Input: dimensioned drawing with shaded views. Units: mm. Origin: part minimum x, y, z. A direction names the side the tool comes from. Round coordinates to 2 decimals unless told otherwise and drop trailing zeros. Loops run counter-clockwise (first coordinate to the right, second up) from the corner with the lowest first, then second, coordinate; pieces in that order, holes last. Notation, with made-up numbers: (4.5, -35.5) -> (10.5, -35.5) arc R13 ccw to (10.5, -18.5) -> close; hole circle Ø3 at (48, 67.5). An arc over 180 degrees is marked (long way). Answer as a JSON object with one key per item and string values.
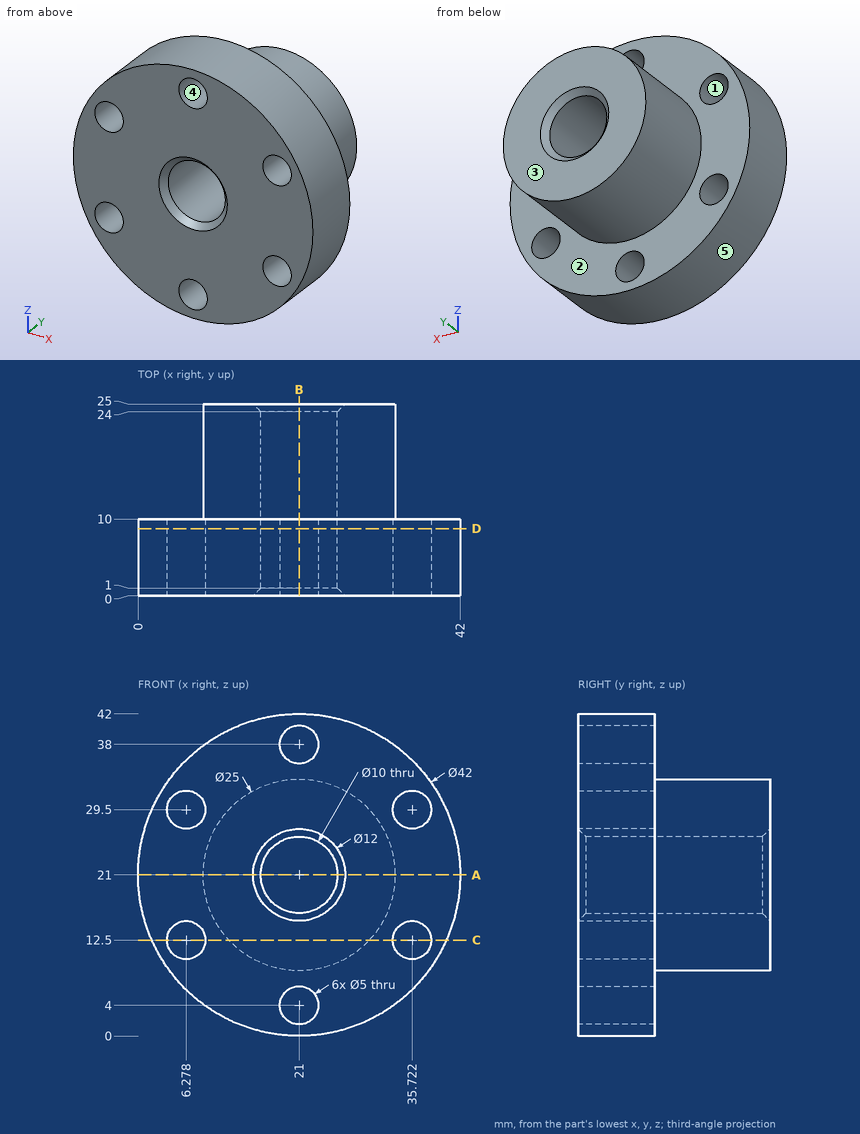
1) Section A-A, the plane z = 21. Output: boundary loops of the cut face in (x, y), plus the area to 3 significant figures.
Output:
{"outline": "(0, 0) -> (15, 0) -> (16, 1) -> (16, 24) -> (15, 25) -> (8.5, 25) -> (8.5, 10) -> (0, 10) -> close; (26, 1) -> (27, 0) -> (42, 0) -> (42, 10) -> (33.5, 10) -> (33.5, 25) -> (27, 25) -> (26, 24) -> close", "area": "543 mm^2"}
2) Ray query, probe 1 along X at (y, z) = (2.5, 12.5); probe 2 along Z at (x, y) = (8, 1.25); probe 3 along Y at (x, z) = (17, 6). Return the intervals inside material, ascending.
Output:
{"probe 1": "x = 1.8 to 3.78, 8.78 to 33.22, 38.22 to 40.2", "probe 2": "z = 4.51 to 10.69, 14.31 to 27.69, 31.31 to 37.49", "probe 3": "y = 0 to 10"}
3) Section B-B, the plane x = 21. Output: boundary loops of the cut face in (y, z).
Output:
{"outline": "(0, 0) -> (10, 0) -> (10, 1.5) -> (0, 1.5) -> close; (0, 6.5) -> (10, 6.5) -> (10, 8.5) -> (25, 8.5) -> (25, 15) -> (24, 16) -> (1, 16) -> (0, 15) -> close; (0, 27) -> (1, 26) -> (24, 26) -> (25, 27) -> (25, 33.5) -> (10, 33.5) -> (10, 35.5) -> (0, 35.5) -> close; (0, 40.5) -> (10, 40.5) -> (10, 42) -> (0, 42) -> close"}
4) Section D-D, the plane y = 8.75. Output: boundary loops of the cut face in (x, z).
Output:
{"outline": "circle Ø42 at (21, 21); hole circle Ø5 at (6.28, 12.5); hole circle Ø5 at (6.28, 29.5); hole circle Ø10 at (21, 21); hole circle Ø5 at (21, 4); hole circle Ø5 at (21, 38); hole circle Ø5 at (35.72, 12.5); hole circle Ø5 at (35.72, 29.5)"}
5) Section C-C, the plane z = 12.5. Output: boundary loops of the cut face in (x, y) (1 decimal), plus the area to 3 significant figures.
Output:
{"outline": "(1.8, 0) -> (3.8, 0) -> (3.8, 10) -> (1.8, 10) -> close; (8.8, 0) -> (33.2, 0) -> (33.2, 10) -> (30.2, 10) -> (30.2, 25) -> (11.8, 25) -> (11.8, 10) -> (8.8, 10) -> close; (38.2, 0) -> (40.2, 0) -> (40.2, 10) -> (38.2, 10) -> close", "area": "559 mm^2"}
6) Reachability of the marked faces 1 and 2 from +Z, -Z, +X, -X, +Y, -Y: full face, straight path, thin tool, end or side. Return the list, or none.
Output:
{"face 1": "+Y, -Y", "face 2": "+Y"}
7) Contact query for flat-ended pins moving along their axis: P1, Ø4, axis at y = 6, z = 5, coming from the +X side; P2, Ø5, axis at x = 9, z = 5.5, coming from the +Y side; P3, Ø1.5, axis at x = 15.5, y = 12, coming from the -Z side. Output: stop coordinate, or through.
Output:
{"P1": "stops at x = 36.65", "P2": "stops at y = 10", "P3": "stops at z = 9.44"}
8) Draft query along Z for the marked faces 3, 4 and 5. Return one class per face: +Z half, -Z half, draft (parallel to the pull), parting line (faces both ways), or undercut.
Output:
{"face 3": "draft", "face 4": "undercut", "face 5": "parting line"}
